from build123d import *

# Parameters (mm, degrees)
SKETCH1_W          = 19.05
SKETCH1_H          = 2.413
CHAMFER1_SIZE      = 0.79375
CUT_EXTRUDE2_DEPTH = 1.79578
SKETCH6_R          = 1.833087105
CUT_EXTRUDE3_DEPTH = 1.79578
CUT_EXTRUDE3_TAPER = 45


with BuildPart() as part:
    # Sketch1 → Revolve1 (revolve)
    with BuildSketch(Plane(origin=(0, 0, 0), x_dir=(0, 0, -1), z_dir=(1, 0, 0))):
        with Locations((12.0904, 1.2065)):
            Rectangle(SKETCH1_W, SKETCH1_H)
    revolve(axis=Axis((0, 0, -21.6154), (0, 0, 1)))

    # Chamfer1
    chamfer1_edges = [part.edges().sort_by_distance(p)[0] for p in [
        (0, -2.413, -21.6154),
    ]]
    chamfer(chamfer1_edges, length=CHAMFER1_SIZE)

    # Sketch7 → Revolve2 (revolve)
    with BuildSketch(Plane(origin=(0, 0, 0), x_dir=(0, 0, -1), z_dir=(1, 0, 0)), mode=Mode.PRIVATE) as revolve2_sk:
        with BuildLine():
            Line((2.18059, 4.5847), (2.5654, 4.5847))
            Line((2.5654, 4.5847), (2.5654, 0))
            Line((2.5654, 0), (0, 0))
            Line((0, 0), (0, 2.413))
            ThreePointArc((0, 2.413), (0.925030326, 3.664791196), (2.18059, 4.5847))
        make_face()
    revolve(revolve2_sk.sketch.rotate(Axis((0, 0, 0), (0, 0, -1)), 180), axis=Axis((0, 0, 0), (0, 0, -1)))

    # Sketch5 → Cut-Extrude2 (cut)
    with BuildSketch(Plane.XY):
        Polygon((1.5875, -0.916543552), (1.5875, 0.916543552), (0, 1.833087105), (-1.5875, 0.916543552), (-1.5875, -0.916543552), (0, -1.833087105), align=None)
    extrude(amount=-CUT_EXTRUDE2_DEPTH, mode=Mode.SUBTRACT)

    # Sketch6 → Cut-Extrude3 (cut)
    with BuildSketch(Plane.XY):
        Circle(SKETCH6_R)
    extrude(amount=-CUT_EXTRUDE3_DEPTH, taper=CUT_EXTRUDE3_TAPER, mode=Mode.SUBTRACT)


solid = part.part
CAD build for the part. Positions are in the model's coordinates, mm. A direction names the side the tool comes from. Coordinates: 2 decimals unless noted, no trailing zeros. Loops run counter-clockwise (first coordinate to the right, second up) from the corner with the lowest first, then second, coordinate; pieces in that order, holes last. Notation, with made-up numbers: (-20, -17.5) - (-8, -17.5) arc R19 cw to (-8, -8.5) - close; hole circle Ø5 at (33, -32). An arc over 180 degrees is marked (long way). Write item = value, one per line. Start each with the question number.
Q1. Which spindle directions (+Z, -Z, +X, -X, +Y, -Y) get a long thin tool onto all of the face, cutting with end or side? Do faces 1 (the flat face through (0, 0, -1.796)), 2 (the flat face through (-2, 0, 0)), 3 (the cylindrical face through (1.468, -1.915, -11.821)). Say none if no direction does.
Q2. Cut at C-C, the plane x = 3.25. List the corners of the cut face in (y, z).
Q3. Cut at D-D, the plane y = -3. List the corners of the cut face in (x, z), then the cut area to 3 significant figures.
Q4. Cut at B-B, the plane z = -10. List the corners of the cut face in (x, y).
Q5. Drill centre lines: L1, parallel to Y at x = -1.5, z = -1.5; L2, parallel to X at y = 0.5, z = -1.75; L3, parallel to X at y = -1.5, z = -1.25. Where is each one in solid material? Low to high.
Q6. Flat gauge pins, fed straight in: pin 1 Ø1 at (x, y) = (-0.5, 0) entering from +Z; pin 2 Ø1.4 at (y, z) = (0, -1) entering from +X; pin 3 Ø0.9 at (y, z) = (0, -0.5) entering from -X. Where does each tip first touch, or does it go through?
Q7. Cut at A-A, the plane y = 0. List the corners of the cut face in (x, z), then the cut area to 3 significant figures.
Q8. Pull direction X, two halves, no side cores. Call faces 4 (the cylindrical face through (4.476, 0.994, -2.376)), 5 (the flat face through (2, -2, -2.565)), 6 (the conical face through (-0.865, -1.473, -0.125)): pulls with the +X half, pulls with the -X half, needs draft (parallel to the pull), parting line crosses it, or undercut.
Computed:
q1.face_1 = +Z
q1.face_2 = +Z, +X, -X, +Y, -Y
q1.face_3 = -Z
q2.outline = (-3.23, -2.57) - (3.23, -2.57) - (3.23, -2.18) arc R4.02 ccw to (-3.23, -2.18) - close
q3.outline = (-3.47, -2.57) - (3.47, -2.57) - (3.47, -2.18) arc R4.21 ccw to (-3.47, -2.18) - close
q3.area = 11.5 mm²
q4.outline = circle Ø4.83 at (0, 0)
q5.L1 = -3.88 to -0.97, 0.97 to 3.88
q5.L2 = -4.3 to -1.59, 1.59 to 4.3
q5.L3 = -3.67 to -0.58, 0.58 to 3.67
q6.pin_1 = -1.8
q6.pin_2 = 4.3
q6.pin_3 = -3.69
q7.outline = (-4.58, -2.57) - (-2.41, -2.57) - (-2.41, -20.82) - (-1.62, -21.62) - (1.62, -21.62) - (2.41, -20.82) - (2.41, -2.57) - (4.58, -2.57) - (4.58, -2.18) arc R5.17 ccw to (2.41, 0) - (1.83, 0) - (1.59, -0.25) - (1.59, -1.8) - (-1.59, -1.8) - (-1.59, -0.25) - (-1.83, 0) - (-2.41, 0) arc R5.17 ccw to (-4.58, -2.18) - close
q7.area = 105 mm²
q8.face_4 = parting line crosses it
q8.face_5 = needs draft
q8.face_6 = undercut
